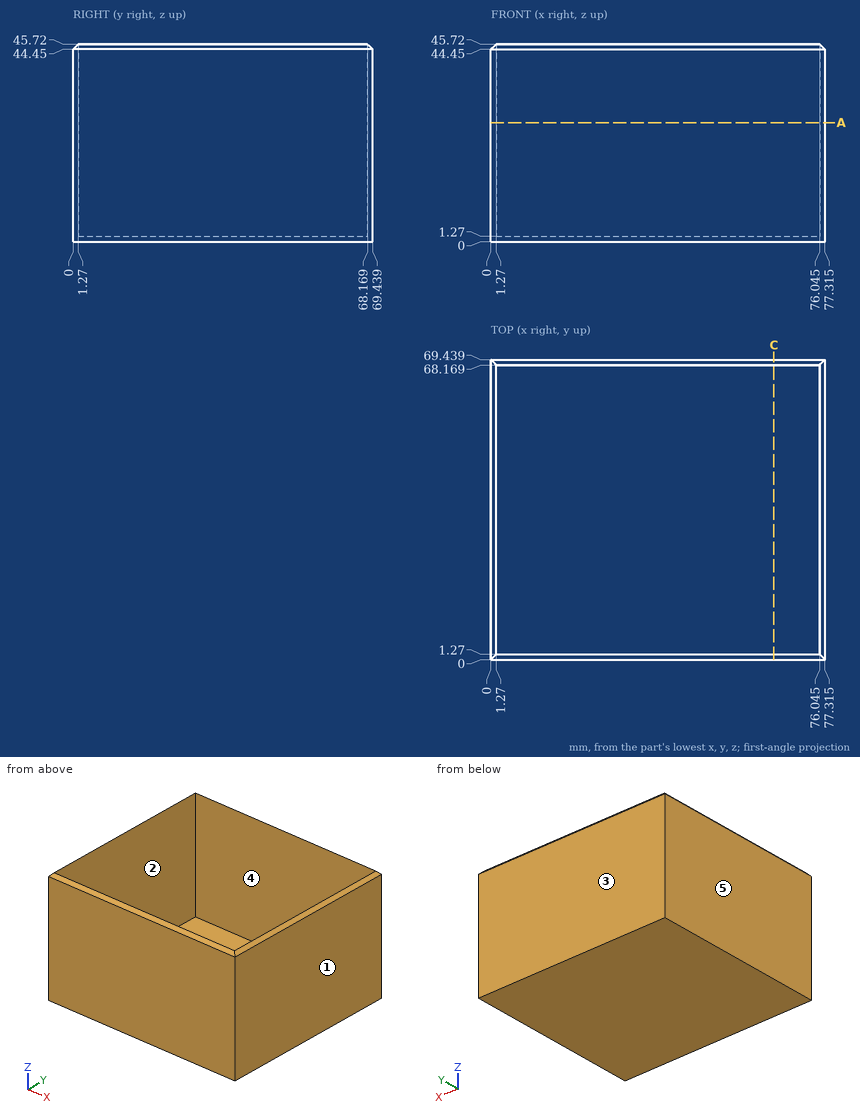
Print and shaded views of the part. All mm, measured from the part's lowest x, y and z. A direction names the side the tool comes from. Round coordinates to 2 decimals unless told otherwise and drop trailing zeros. Write each loop counter-clockwise with the first axis right and the second up, starting at its lowest first coordinate (ties: lowest second). Pieces come first, ordered by that corner, then holes. Notation, with made-up numbers: (-6.75, 23) -> (32.25, 23) arc R15 cw to (32.25, 40) -> close; hole circle Ø8 at (35, -19). An arc over 180 degrees is marked (long way). Return JSON: item names as keys, results as strings. Group by question number.
Q1. Saw through at A-A on z = 27.5. Write the cut outline in (x, y) (1 decimal).
Q2. Pin check, flat tip, straight feed: pin 1 (20 mm diameter, centred on x = 29, y = 35, fed in from +Z). Stop position of the tip, or through.
Q3. Mould opens along Y. For the marked faces 3, 4 and 5 say: pulls with the +Y half, pulls with the -Y half, needs draft (parallel to the pull), parting line crosses it, or undercut.
Q4. Saw through at C-C on x = 65.5. Write the cut outline in (y, z).
Q5. Which spindle directions (+Z, -Z, +X, -X, +Y, -Y) get a long thin tool onto all of the face, cutting with end or side? Do the marked faces 1 and 2. Say none if no direction does.
Q6. Probe L1, parallel to Y at x = 46, z = 38.5; L2, parallel to X at y = 58.5, z = 15 (1 decimal); L3, parallel to Z at x = 51.5, y = 56. List the from-to ranges inside material, lowest first. Write a range as [from, to].
Answer:
{
 "1": {"outline": "(0, 0) -> (77.3, 0) -> (77.3, 69.4) -> (0, 69.4) -> close; hole (1.3, 1.3) -> (76, 1.3) -> (76, 68.2) -> (1.3, 68.2) -> close"},
 "2": {"pin 1": "z = 1.27"},
 "3": {"face 3": "pulls with the +Y half", "face 4": "undercut", "face 5": "needs draft"},
 "4": {"outline": "(0, 0) -> (69.44, 0) -> (69.44, 44.45) -> (68.17, 45.72) -> (68.17, 1.27) -> (1.27, 1.27) -> (1.27, 45.72) -> (0, 44.45) -> close"},
 "5": {"face 1": "+Z, -Z, +X, +Y, -Y", "face 2": "+Z"},
 "6": {"L1": "[0, 1.27], [68.17, 69.44]", "L2": "[0, 1.3], [76, 77.3]", "L3": "[0, 1.27]"}
}
